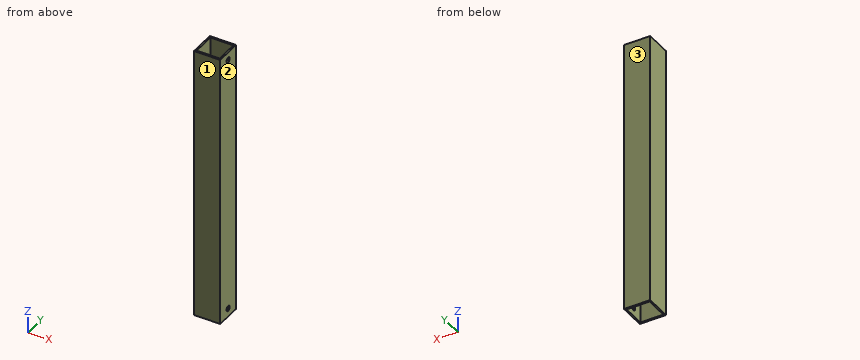
Autodesk Inventor part; units mm, degrees
ref_plane "YZ Plane" through (0, 0, 0) normal (1, 0, 0) x (0, 1, 0)
ref_plane "XZ Plane" through (0, 0, 0) normal (0, 1, 0) x (-1, 0, 0)
ref_plane "XY Plane" through (0, 0, 0) normal (0, 0, 1) x (1, 0, 0)
sketch "Sketch1" plane through (0, 0, 0) normal (0, 0, 1) x (1, 0, 0)
  line L0 (12.7, -12.7) -> (-12.7, -12.7)
  line L1 (-12.7, -12.7) -> (-12.7, 12.7)
  line L2 (-12.7, 12.7) -> (12.7, 12.7)
  line L3 (12.7, 12.7) -> (12.7, -12.7)
  line L4 (12.7, -12.7) -> (-12.7, 12.7) construction
  line L5 (-12.7, -12.7) -> (12.7, 12.7) construction
  line L6 (11.049, 11.049) -> (-11.049, 11.049)
  line L7 (-11.049, 11.049) -> (-11.049, -11.049)
  line L8 (-11.049, -11.049) -> (11.049, -11.049)
  line L9 (11.049, -11.049) -> (11.049, 11.049)
  line L10 (11.049, 11.049) -> (-11.049, -11.049) construction
  line L11 (-11.049, 11.049) -> (11.049, -11.049) construction
  point P0 (0, 0)
  dimension "d0" = 25.4
  dimension "d1" = 25.4
  dimension "d2" = 1.651
  dimension "d3" = 1.651
extrude "Extrusion1" add sketch "Sketch1" along normal blind 266.7
sketch "Sketch2" plane through (12.7, -12.7, 0) normal (1, 0, 0) x (0, 0, -1)
  circle A0 centre (-8.1788, 12.7) radius 2.54
  circle A1 centre (-259.08, 12.7) radius 2.54
  line L0 (0, 25.4) -> (0, 0)
  line L1 (-266.7, 0) -> (-266.7, 25.4)
  line L2 (0, 0) -> (-266.7, 0)
  point P0 (0, 12.7)
  dimension "d6" = 250.9012
  dimension "d7" = 5.08
  dimension "d8" = 5.08
  dimension "d15" = 12.7
  dimension "d16" = 12.7
  dimension "d17" = 7.62
extrude "Extrusion2" cut sketch "Sketch2" against normal blind 2.54
equation "\"d3\" = d2"
equation "\"d8\" = d7"
properties part number "push bar"
Verification items for the finished model (mm, model axes). Face numbers are marked on the shaded views. Give positions to 0.01 mm unless a question says otherwise; leave off trailing zeros. Write each loop counter-clockwise with the first axis right and the second up, starting at its lowest first coordinate (ties: lowest second). Pieces come first, ordered by that corner, then holes.
(1) Mould release check, pull along Y, two halves, no side actions. Record for the marked faces 1, 2 and 3: +Y half, -Y half, draft (parallel to the pull), parting line (faces both ways), or undercut.
(2) Cross-section at B-B (z = 229). Enter the section's corners in (x, y), plus the area to 3 significant figures.
(3) Cross-section at C-C (x = 3.5). Enter the section's corners in (y, z).
(4) Cross-section at D-D (z = 259.08). Enter the section's corners in (x, y).
(5) Material ranges on line 1 (X direction, y = -1, z = 187); line 2 (Y direction, x = 12.1, z = 259.08), recorded low to high.
(6) Cross-section at A-A (y = 0). Enter the section's corners in (x, z), plus the area to 3 significant figures.
Worked out:
1. face 1: -Y half
1. face 2: draft
1. face 3: +Y half
2. outline: (-12.7, -12.7) - (12.7, -12.7) - (12.7, 12.7) - (-12.7, 12.7) - close; hole (-11.05, -11.05) - (11.05, -11.05) - (11.05, 11.05) - (-11.05, 11.05) - close
2. area: 157 mm2
3. outline: (-12.7, 0) - (-11.05, 0) - (-11.05, 266.7) - (-12.7, 266.7) - close; (11.05, 0) - (12.7, 0) - (12.7, 266.7) - (11.05, 266.7) - close
4. outline: (-12.7, -12.7) - (12.7, -12.7) - (12.7, -2.54) - (11.05, -2.54) - (11.05, -11.05) - (-11.05, -11.05) - (-11.05, 11.05) - (11.05, 11.05) - (11.05, 2.54) - (12.7, 2.54) - (12.7, 12.7) - (-12.7, 12.7) - close
5. line 1: x = -12.7 to -11.05, 11.05 to 12.7
5. line 2: y = -12.7 to -2.54, 2.54 to 12.7
6. outline: (-12.7, 0) - (-11.05, 0) - (-11.05, 266.7) - (-12.7, 266.7) - close; (11.05, 0) - (12.7, 0) - (12.7, 5.64) - (11.05, 5.64) - close; (11.05, 10.72) - (12.7, 10.72) - (12.7, 256.54) - (11.05, 256.54) - close; (11.05, 261.62) - (12.7, 261.62) - (12.7, 266.7) - (11.05, 266.7) - close
6. area: 864 mm2
